Geometry: see drawing. Coordinates: mm, zero at the bounding-box minimum. Round coordinates to 2 decimals unless told otherwise and drop trailing zeros. Write each loop counter-clockwise with the first axis right and the second up, starting at its lowest first coordinate (ties: lowest second). Pieces come first, ordered by that corner, then holes. Notation, with made-up numbers: (45, 68) -> (68, 68) arc R22 ccw to (68, 76) -> close; hole circle Ø7 at (75, 67.25). An arc over 180 degrees is marked (long way). Write item = value, one per line.
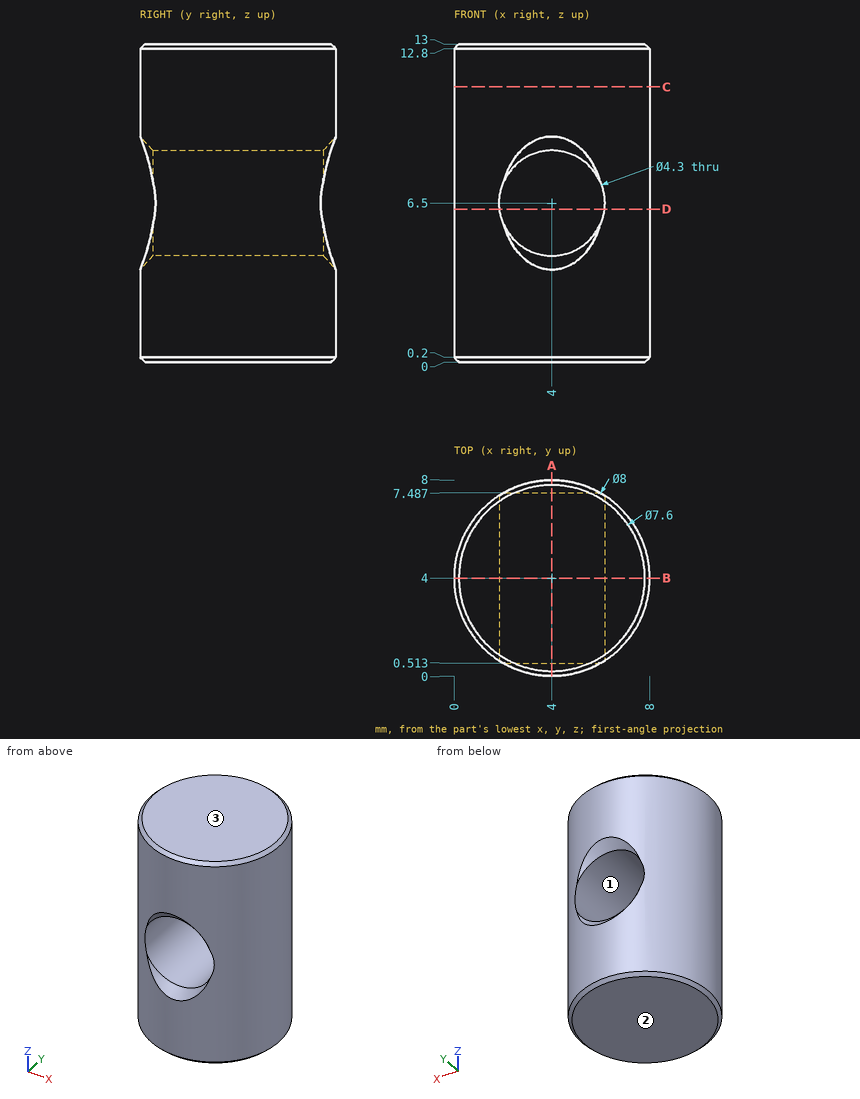
1) Cut plane A-A (x = 4). Return the cut outline in (y, z).
Solutions:
outline = (0, 0.2) -> (0.2, 0) -> (7.8, 0) -> (8, 0.2) -> (8, 3.78) -> (7.49, 4.35) -> (0.51, 4.35) -> (0, 3.78) -> close; (0, 9.22) -> (0.51, 8.65) -> (7.49, 8.65) -> (8, 9.22) -> (8, 12.8) -> (7.8, 13) -> (0.2, 13) -> (0, 12.8) -> close
2) Draft query along Z for the marked faces 1, 2 and 3. Return one class per face: +Z half, -Z half, draft (parallel to the pull), parting line (faces both ways), or undercut.
Solutions:
face_1 = undercut
face_2 = -Z half
face_3 = +Z half
3) First-contact query: P1, Ø4, axis at x = 1.5, z = 1.5, coming from the -Y side; P2, Ø1, axis at y = 1.5, z = 10.5, coming from the -X side (1 decimal). Flat tips, straight axial feed; report the tip coordinate or a pass-through.
Solutions:
P1 = 0.03
P2 = 0.5
4) Cut plane D-D (z = 6.25). Return the cut outline in (x, y) (1 decimal).
Solutions:
outline = (1.9, 0.6) -> (1.9, 7.4) arc R4 ccw to start; (6.1, 0.6) arc R4 ccw to (6.1, 7.4) -> close
5) Line query: L1, parallel to X at y = 2.75, z = 6.5; L2, parallel to Z at x = 3.5, y = 4; L3, parallel to Z at x = 2.25, y = 2.5. Output: solid intervals per line, ascending. Write a range as from..to.
Solutions:
L1 = 0.2..1.85, 6.15..7.8
L2 = 0..4.41, 8.59..13
L3 = 0..5.25, 7.75..13
6) Cut plane C-C (z = 11.25). Return the cut outline in (x, y).
Solutions:
outline = circle Ø8 at (4, 4)
7) Cut plane B-B (y = 4). Return the cut outline in (x, z).
Solutions:
outline = (0, 0.2) -> (0.2, 0) -> (7.8, 0) -> (8, 0.2) -> (8, 12.8) -> (7.8, 13) -> (0.2, 13) -> (0, 12.8) -> close; hole circle Ø4.3 at (4, 6.5)
